```python
from build123d import *

# Parameters (mm, degrees)
PARKING_DEPTH       = 10
PARKINGS_COUNT      = 3
PARKINGS_PITCH      = 90
RIGHTWALL_DEPTH     = 5
LASERHOLE_REACH     = 351.321
SKETCH2_W           = 20
SKETCH2_H           = 20
SKETCH5_W           = 420
SKETCH5_H           = 130
PARKINGBOTTOM_DEPTH = 20
CARTBOTTOM_DEPTH    = 425
SKETCH9_R           = 5
THREADEDROD_DEPTH   = 300


with BuildPart() as part:
    # SingleLot → Parking (new body)
    with BuildSketch(Plane(origin=(0, 0, 0), x_dir=(1, 0, 0), z_dir=(0, 1, 0))):
        Polygon((5, 70), (0, 70), (0, 200), (90, 200), (90, 70), (85, 70), (85, 190), (5, 190), align=None)
    parking = extrude(amount=PARKING_DEPTH)

    # Parkings: Parking ×3
    with Locations(*[(i * PARKINGS_PITCH, 0, 0) for i in range(1, PARKINGS_COUNT)]):
        add(parking)

    # Wall → RightWall (add)
    with BuildSketch(Plane(origin=(270, 0, 0), x_dir=(0, 0, -1), z_dir=(1, 0, 0))):
        Polygon((0, 65), (0, 80), (200, 80), (200, 0), (200, -20), (0, -20), (0, 0), (0, 55), (5, 55), (5, 65), align=None)
    extrude(amount=RIGHTWALL_DEPTH)

    # Sketch2 → LaserHole (cut, up to next)
    with BuildSketch(Plane(origin=(275, 0, 0), x_dir=(0, 0, -1), z_dir=(1, 0, 0)), mode=Mode.PRIVATE) as laserhole_sk1:
        with Locations((70, 30)):
            Rectangle(SKETCH2_W, SKETCH2_H)
    laserhole_tool1 = extrude(laserhole_sk1.sketch, amount=-LASERHOLE_REACH, mode=Mode.PRIVATE) & part.part
    add(laserhole_tool1.solids().sort_by_distance((275, 30, -70))[0], mode=Mode.SUBTRACT)

    # Sketch5 → ParkingBottom (add)
    with BuildSketch(Plane.XZ):
        with Locations((60, -135)):
            Rectangle(SKETCH5_W, SKETCH5_H)
    extrude(amount=PARKINGBOTTOM_DEPTH)

    # Sketch8 → CartBottom (add)
    with BuildSketch(Plane.ZY.offset(150)):
        with BuildLine():
            Line((-70, -20), (0, -20))
            Line((0, -20), (0, -17))
            ThreePointArc((0, -17), (-3.535533906, -15.535533906), (-5, -12))
            Line((-5, -12), (-45, -12))
            ThreePointArc((-45, -12), (-50, -17), (-55, -12))
            Line((-55, -12), (-70, -12))
            Line((-70, -12), (-70, -20))
        make_face()
    extrude(amount=-CARTBOTTOM_DEPTH)

    # Mirror8: part across plane


with BuildPart() as part_1:
    add(part.part)
    add(part.part.mirror(Plane.XY))

    # Sketch9 → ThreadedRod (add)
    with BuildSketch(Plane(origin=(0, 0, 0), x_dir=(1, 0, 0), z_dir=(0, 1, 0))):
        with Locations(Location((-130, 90, 0), (0, 0, 270))):
            Circle(SKETCH9_R)
        with Locations(Location((-20, 180, 0), (0, 0, 270))):
            Circle(SKETCH9_R)
    extrude(amount=THREADEDROD_DEPTH)


solid = part_1.part
```
The model under review builds one solid part; all positions refer to its coordinate system, in mm. A direction names the side the tool comes from. Round coordinates to 2 decimals unless told otherwise and drop trailing zeros. Loops run counter-clockwise (first coordinate to the right, second up) from the corner with the lowest first, then second, coordinate; pieces in that order, holes last.
Item 1: For faces 3 (the face through (-150, -17, 3)), 4 (the face through (265, 5, 129)), 5 (the face through (57, -12, 25)), list the 3-axis set-ups (+Z, -Z, +X, -X, +Y, -Y) from which the entire face can be reached by the end or side of a thin tool; tool diameter is ignored.
Determined:
face 3: +Z, -Z, -X, +Y, -Y
face 4: +Y
face 5: -X, +Y
Item 2: Mouldability with a two-part tool opening along Z and no side actions: class faces 1 (the face through (85, 5, 129)), 2 (the face through (0, 5, 134)) as released by +Z, released by -Z, zero draft, split by the parting line, or undercut.
Determined:
face 1: undercut
face 2: zero draft
Item 3: Take a section at D-D (z = -18). Write out the cut boundary in (x, y).
Determined:
outline: (-150, -20) - (275, -20) - (275, 80) - (270, 80) - (270, -12) - (-150, -12) - close
Item 4: Take a section at B-B (z = 174). Write out the cut boundary in (x, y).
Determined:
outline: (-150, -20) - (275, -20) - (275, 80) - (270, 80) - (270, 10) - (265, 10) - (265, 0) - (185, 0) - (185, 10) - (175, 10) - (175, 0) - (95, 0) - (95, 10) - (85, 10) - (85, 0) - (5, 0) - (5, 10) - (0, 10) - (0, 0) - (-150, 0) - close
Item 5: For line 1 (X direction, y = 51, z = -1.5); line 2 (Y direction, x = -28, z = -110.5); line 3 (Y direction, x = 199.5, z = 1), list the stretches that pass through material, from the lowest coordinate up.
Determined:
line 1: x = 270 to 275
line 2: y = -20 to 0
line 3: y = -20 to -16.9
Item 6: Clearance check with flat-ended pins moving along their axes: pin 1 Ø3 at (y, z) = (7.5, -115.5) entering from -X; pin 2 Ø2 at (x, z) = (-41, -63.5) entering from +Y; pin 3 Ø5.5 at (x, z) = (272, -73.5) entering from +Y. State where each tip first meets the part, or that it passes through.
Determined:
pin 1: stops at x = 0
pin 2: stops at y = -12
pin 3: stops at y = 80
Item 7: Take a section at C-C (y = 243.5). Write out the cut boundary in (x, z), then the cut area to 3 significant figures.
Determined:
outline: circle Ø10 at (-130, -90); circle Ø10 at (-20, -180)
area: 157 mm2
Item 8: Take a section at A-A (x = 229). Write out the cut boundary in (y, z).
Determined:
outline: (-20, -200) - (10, -200) - (10, -190) - (0, -190) - (0, -70) - (-12, -70) - (-12, -55) arc R5 cw to (-12, -45) - (-12, -5) arc R5 cw to (-12, 5) - (-12, 45) arc R5 cw to (-12, 55) - (-12, 70) - (0, 70) - (0, 190) - (10, 190) - (10, 200) - (-20, 200) - close
